Geometry check sheet. Reference: the model listing, model coordinates, mm. A direction names the side the tool comes from. Give positions to 0.01 mm unless a question says otherwise; leave off trailing zeros. Write each loop counter-clockwise with the first axis right and the second up, starting at its lowest first coordinate (ties: lowest second). Pieces come first, ordered by that corner, then holes. Notation, with made-up numbers: M 58,-1 L 109,-1 A25 cw 109,11 Z; hole C -4,62 d10. An arc over 180 degrees is marked long. Use one line per item in the form item = value. Start each with the question number.
```python
from build123d import *

# Parameters (mm, degrees)
SKETCH_1_W          = 200
SKETCH_1_H          = 120
EXTRUDE_1_DEPTH     = 3
SKETCH_2_R          = 1.525
CUT_EXTRUDE_1_DEPTH = 3
SKETCH_3_W          = 120
SKETCH_3_H          = 40
CUT_EXTRUDE_2_DEPTH = 3
CUT_EXTRUDE_3_DEPTH = 10
SKETCH_5_W          = 200
SKETCH_5_H          = 20
EXTRUDE_2_DEPTH     = 3
SKETCH_7_R          = 1.525
CUT_EXTRUDE_4_DEPTH = 4
SKETCH_14_R         = 2.025
CUT_EXTRUDE_5_DEPTH = 4
SKETCH_15_R         = 2.025
CUT_EXTRUDE_6_DEPTH = 4
FILLET_1_R          = 3


with BuildPart() as part:
    # 草图1 → 凸台-拉伸1 (new body)
    with BuildSketch(Plane(origin=(0, 0, 0), x_dir=(1, 0, 0), z_dir=(0, 1, 0))):
        Rectangle(SKETCH_1_W, SKETCH_1_H)
    extrude(amount=EXTRUDE_1_DEPTH)

    # 草图2 → 切除-拉伸1 (cut)
    with BuildSketch(Plane(origin=(0, 3, 0), x_dir=(1, 0, 0), z_dir=(0, 1, 0))):
        with Locations((67.5, 54.2)):
            Circle(SKETCH_2_R)
        with Locations((87.5, 54.2)):
            Circle(SKETCH_2_R)
        with Locations((67.5, -54.2)):
            Circle(SKETCH_2_R)
        with Locations((87.5, -54.2)):
            Circle(SKETCH_2_R)
        with Locations((-87.5, -54.2)):
            Circle(SKETCH_2_R)
        with Locations((-67.5, -54.2)):
            Circle(SKETCH_2_R)
        with Locations((-87.5, 54.2)):
            Circle(SKETCH_2_R)
        with Locations((-67.5, 54.2)):
            Circle(SKETCH_2_R)
    extrude(amount=-CUT_EXTRUDE_1_DEPTH, mode=Mode.SUBTRACT)

    # 草图3 → 切除-拉伸2 (cut)
    with BuildSketch(Plane(origin=(0, 3, 0), x_dir=(1, 0, 0), z_dir=(0, 1, 0))):
        with Locations((0, 60)):
            Rectangle(SKETCH_3_W, SKETCH_3_H)
    extrude(amount=-CUT_EXTRUDE_2_DEPTH, mode=Mode.SUBTRACT)

    # 草图4 → 切除-拉伸3 (cut)
    with BuildSketch(Plane(origin=(0, 3, 0), x_dir=(1, 0, 0), z_dir=(0, 1, 0))):
        with BuildLine():
            Line((-80, 30), (80, 30))
            ThreePointArc((80, 30), (85, 25), (80, 20))
            Line((80, 20), (-80, 20))
            ThreePointArc((-80, 20), (-85, 25), (-80, 30))
        make_face()
        with BuildLine():
            Line((-80, 9), (80, 9))
            ThreePointArc((80, 9), (85, 4), (80, -1))
            Line((80, -1), (-80, -1))
            ThreePointArc((-80, -1), (-85, 4), (-80, 9))
        make_face()
        with BuildLine():
            Line((-80, -12), (80, -12))
            ThreePointArc((80, -12), (85, -17), (80, -22))
            Line((80, -22), (-80, -22))
            ThreePointArc((-80, -22), (-85, -17), (-80, -12))
        make_face()
        with BuildLine():
            Line((-80, -33), (80, -33))
            ThreePointArc((80, -33), (85, -38), (80, -43))
            Line((80, -43), (-80, -43))
            ThreePointArc((-80, -43), (-85, -38), (-80, -33))
        make_face()
    extrude(amount=-CUT_EXTRUDE_3_DEPTH, mode=Mode.SUBTRACT)

    # 草图5 → 凸台-拉伸2 (add)
    with BuildSketch(Plane(origin=(0, 3, 0), x_dir=(1, 0, 0), z_dir=(0, 1, 0))):
        with Locations((0, -70)):
            Rectangle(SKETCH_5_W, SKETCH_5_H)
    extrude(amount=-EXTRUDE_2_DEPTH)

    # 草图7 → 切除-拉伸4 (cut, through all)
    with BuildSketch(Plane(origin=(0, 3, 0), x_dir=(1, 0, 0), z_dir=(0, 1, 0))):
        with Locations((-87.5, -75.8)):
            Circle(SKETCH_7_R)
        with Locations((-67.5, -75.8)):
            Circle(SKETCH_7_R)
    cut_extrude_4 = extrude(amount=-CUT_EXTRUDE_4_DEPTH, mode=Mode.SUBTRACT)

    # 镜向1: 切除-拉伸4 across plane
    add(cut_extrude_4.mirror(Plane(origin=(0, 0, 0), x_dir=(0, 0, 1), z_dir=(1, 0, 0))), mode=Mode.SUBTRACT)

    # 草图12 → 孔2 (revolve, cut)
    with BuildSketch(Plane(origin=(-77.5, 0, 65), x_dir=(0, 0, -1), z_dir=(1, 0, 0))):
        Polygon((0, 0), (0, 3), (2, 3), (2, 2), (4, 0), align=None)
    hole_wizard_2 = revolve(axis=Axis((-77.5, -6.445314094, 65), (0, 1, 0)), mode=Mode.SUBTRACT)

    # 镜向3: 孔2 across plane
    add(hole_wizard_2.mirror(Plane(origin=(0, 0, 0), x_dir=(0, 0, 1), z_dir=(1, 0, 0))), mode=Mode.SUBTRACT)

    # 草图14 → 切除-拉伸5 (cut, through all)
    with BuildSketch(Plane.XZ):
        with Locations((-70, 6.5)):
            Circle(SKETCH_14_R)
    cut_extrude_5 = extrude(amount=-CUT_EXTRUDE_5_DEPTH, mode=Mode.SUBTRACT)

    # 镜向4: 切除-拉伸5 across plane
    add(cut_extrude_5.mirror(Plane(origin=(0, 0, 0), x_dir=(0, 0, 1), z_dir=(1, 0, 0))), mode=Mode.SUBTRACT)

    # 草图15 → 切除-拉伸6 (cut, through all)
    with BuildSketch(Plane.XZ):
        with Locations((0, 27.5)):
            Circle(SKETCH_15_R)
    extrude(amount=-CUT_EXTRUDE_6_DEPTH, mode=Mode.SUBTRACT)

    # 圆角1
    fillet_1_edges = [part.edges().sort_by_distance(p)[0] for p in [
        (-100, 1.5, 80),
        (100, 1.5, 80),
        (60, 1.5, -60),
        (-60, 1.5, -60),
        (-60, 1.5, -40),
        (60, 1.5, -40),
        (-100, 1.5, -60),
        (100, 1.5, -60),
    ]]
    fillet(fillet_1_edges, radius=FILLET_1_R)


solid = part.part
```
(1) Tool access check on faces 1 (the conical face through (-79.61, 1.87, 65.28)), 2 (the cylindrical face through (-85, 2, -25)). Record the directions out of +Z, -Z, +X, -X, +Y, -Y that give a thin tool (end or side, any length) a straight path to the whole face; none if there is none.
(2) Sectioned sample at A-A, the plane z = 27.5. Record the boundary of the cut face in (x, y) (3 decimals), plus the area to 3 significant figures.
(3) Sectioned sample at C-C, the plane z = 6.5. Record the boundary of the cut face in (x, y) (3 decimals), plus the area to 3 significant figures.
(4) Thickness scan on probe 1 along X at (y, z) = (2.65, 65); probe 2 along X at (y, z) = (1.35, 54.2) (3 decimals); probe 3 along Z at (x, y) = (-77.5, 2.4). Record the ranges inside material, lowest first. Write a range as [from, to].
(5) Draft check along Z on faces 3 (the flat face through (-1, 0, 25)), 4 (the cylindrical face through (85, 2, 38)). Enter one of: released by +Z, released by -Z, zero draft, split by the parting line, or undercut.
(6) Sectioned sample at D-D, the plane x = 14. Record the boundary of the cut face in (y, z), plus the area to 3 significant figures.
(7) Sectioned sample at B-B, the plane x = 77.5. Record the boundary of the cut face in (y, z), plus the area to 3 significant figures.
Numbers:
q1.face_1 = -Y
q1.face_2 = +Y, -Y
q2.outline = M -100,0 L -2.025,0 L -2.025,3 L -100,3 Z; M 2.025,0 L 100,0 L 100,3 L 2.025,3 Z
q2.area = 588 mm2
q3.outline = M -100,0 L -72.025,0 L -72.025,3 L -100,3 Z; M -67.975,0 L 67.975,0 L 67.975,3 L -67.975,3 Z; M 72.025,0 L 100,0 L 100,3 L 72.025,3 Z
q3.area = 576 mm2
q4.probe_1 = [-100, -79.5], [-75.5, 75.5], [79.5, 100]
q4.probe_2 = [-100, -89.025], [-85.975, -69.025], [-65.975, 65.975], [69.025, 85.975], [89.025, 100]
q4.probe_3 = [-60, -30], [-20, -9], [1, 12], [22, 33], [43, 63], [67, 80]
q5.face_3 = zero draft
q5.face_4 = undercut
q6.outline = M 0,-40 L 3,-40 L 3,-30 L 0,-30 Z; M 0,-20 L 3,-20 L 3,-9 L 0,-9 Z; M 0,1 L 3,1 L 3,12 L 0,12 Z; M 0,22 L 3,22 L 3,33 L 0,33 Z; M 0,43 L 3,43 L 3,80 L 0,80 Z
q6.area = 240 mm2
q7.outline = M 0,-60 L 3,-60 L 3,-30 L 0,-30 Z; M 0,-20 L 3,-20 L 3,-9 L 0,-9 Z; M 0,1 L 3,1 L 3,12 L 0,12 Z; M 0,22 L 3,22 L 3,33 L 0,33 Z; M 0,43 L 3,43 L 3,63 L 2,63 L 0,61 Z; M 0,69 L 2,67 L 3,67 L 3,80 L 0,80 Z
q7.area = 284 mm2
